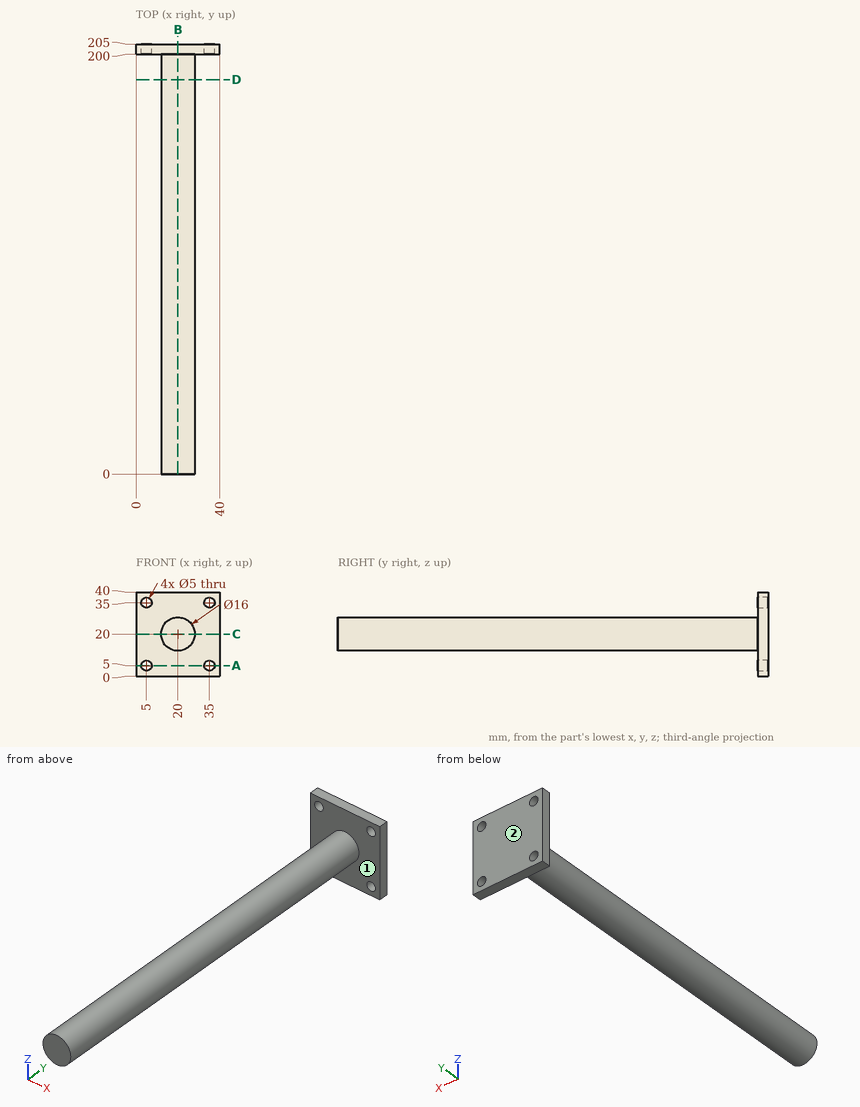
Geometry check sheet. Reference: drawing and pictorial views, mm from the part's lowest x, y, z. A direction names the side the tool comes from. Coordinates: 2 decimals unless noted, no trailing zeros. Write each loop counter-clockwise with the first axis right and the second up, starting at its lowest first coordinate (ties: lowest second). Pieces come first, ordered by that corner, then holes.
Item 1: Access from +Z, -Z, +X, -X, +Y, -Y to the whole of each face (thin tool, end or side, straight path). Record for the marked faces 1 and 2.
Numbers:
face 1: -Y
face 2: +Z, -Z, +X, -X, +Y
Item 2: Cross-section at C-C on z = 20. Record the boundary of the cut face in (x, y).
Numbers:
outline: (0, 200) - (12, 200) - (12, 0) - (28, 0) - (28, 200) - (40, 200) - (40, 205) - (0, 205) - close
Item 3: Scan lines: probe 1 along X at (y, z) = (203.6, 35); probe 2 along Y at (x, z) = (20, 35); probe 3 along Z at (x, y) = (15.5, 69). Record each from-to range of solid material in increasing order.
Numbers:
probe 1: x = 0 to 2.5, 7.5 to 32.5, 37.5 to 40
probe 2: y = 200 to 205
probe 3: z = 13.39 to 26.61
Item 4: Depth check by flat-ended pin: pin 1 Ø5 at (x, z) = (31, 9) entering from -Y; pin 2 Ø6 at (x, y) = (21, 112.5) entering from -Z. Enter the tip coordinate at first touch or a pass-through.
Numbers:
pin 1: stops at y = 200
pin 2: stops at z = 12
Item 5: Cross-section at B-B on x = 20. Record the boundary of the cut face in (y, z), then the cut area to 3 significant figures.
Numbers:
outline: (0, 12) - (200, 12) - (200, 0) - (205, 0) - (205, 40) - (200, 40) - (200, 28) - (0, 28) - close
area: 3,400 mm2
Item 6: Cross-section at D-D on y = 188. Record the boundary of the cut face in (x, z), then the cut area to 3 significant figures.
Numbers:
outline: circle Ø16 at (20, 20)
area: 201 mm2
Item 7: Cross-section at A-A on z = 5. Record the boundary of the cut face in (x, y).
Numbers:
outline: (0, 200) - (2.5, 200) - (2.5, 205) - (0, 205) - close; (7.5, 200) - (32.5, 200) - (32.5, 205) - (7.5, 205) - close; (37.5, 200) - (40, 200) - (40, 205) - (37.5, 205) - close
